Geometry: final body of the model. Coordinates: model frame, mm. Give positions to 0.01 mm unless a question says otherwise; leave off trailing zeros. Loops run counter-clockwise (first coordinate to the right, second up) from the corner with the lowest first, then second, coordinate; pieces in that order, holes last. Notation, with made-up numbers: (61, 5.5) - (81, 5.5) arc R17 cw to (81, 11.5) - close; hole circle Ø10 at (-28.75, 2). An arc over 180 degrees is marked (long way). Use one line per item in the form item = value.
```python
from build123d import *

# Parameters (mm, degrees)
F0_R      = 15.875
F1_DEPTH  = 3.81
F3_DEPTH  = 40.64
F4_DEPTH  = 3.81
F5_DEPTH  = 3.81
F6_DEPTH  = 3.81
F7_DEPTH  = 3.81
F8_DEPTH  = 3.81
F9_DEPTH  = 3.81
F10_DEPTH = 3.81


with BuildPart() as f1:
    # F0 (on Top) → F1 (new body)
    with BuildSketch(Plane.XY):
        with BuildLine():
            Line((-66.04, 50.8), (-88.9, 50.8))
            Line((-88.9, 50.8), (-88.9, 0))
            Line((-88.9, 0), (-69.85, -76.2))
            Line((-69.85, -76.2), (-38.1, -107.95))
            Line((-38.1, -107.95), (0, -107.95))
            Line((0, -107.95), (38.1, -107.95))
            Line((38.1, -107.95), (69.85, -76.2))
            Line((69.85, -76.2), (88.9, 0))
            Line((88.9, 0), (88.9, 50.8))
            Line((88.9, 50.8), (66.04, 50.8))
            Line((66.04, 50.8), (66.04, 1.27))
            Line((66.04, 1.27), (66.04, -36.83))
            Line((66.04, -36.83), (65.8662626902, -36.83))
            ThreePointArc((65.8662626902, -36.83), (47.625, -55.0712626902), (29.3837373098, -36.83))
            Line((29.3837373098, -36.83), (29.21, -36.83))
            Line((29.21, -36.83), (29.21, 1.27))
            Line((29.21, 1.27), (29.21, 50.8))
            Line((29.21, 50.8), (0, 50.8))
            Line((0, 50.8), (-29.21, 50.8))
            Line((-29.21, 50.8), (-29.21, 1.27))
            Line((-29.21, 1.27), (-29.21, -36.83))
            Line((-29.21, -36.83), (-29.3837373098, -36.83))
            ThreePointArc((-29.3837373098, -36.83), (-47.625, -55.0712626902), (-65.8662626902, -36.83))
            Line((-65.8662626902, -36.83), (-66.04, -36.83))
            Line((-66.04, -36.83), (-66.04, 1.27))
            Line((-66.04, 1.27), (-66.04, 50.8))
        make_face()
        with Locations((0, -16.51)):
            Circle(F0_R, mode=Mode.SUBTRACT)
    extrude(amount=F1_DEPTH)

    # F2: F1 across plane


with BuildPart() as f1_1:
    add(f1.part)
    add(f1.part.mirror(Plane.YZ), mode=Mode.INTERSECT)

    # F3 (cut): faces of the model
    f3_faces = [f1_1.faces().sort_by_distance(p)[0] for p in [
        (0, 50.8, 1.905),
        (77.47, 50.8, 1.905),
        (-77.47, 50.8, 1.905),
    ]]
    extrude(f3_faces, amount=-F3_DEPTH, mode=Mode.SUBTRACT)

    # F4 (add): a face of the model
    f4_faces = [f1_1.faces().sort_by_distance(p)[0] for p in [
        (0, -107.95, 1.905),
    ]]
    extrude(f4_faces, amount=F4_DEPTH)

    # F5 (add): a face of the model
    f5_faces = [f1_1.faces().sort_by_distance(p)[0] for p in [
        (-53.975, -92.075, 1.905),
    ]]
    extrude(f5_faces, amount=F5_DEPTH)

    # F6 (add): a face of the model
    f6_faces = [f1_1.faces().sort_by_distance(p)[0] for p in [
        (-79.375, -38.1, 1.905),
    ]]
    extrude(f6_faces, amount=F6_DEPTH)

    # F7 (add): a face of the model
    f7_faces = [f1_1.faces().sort_by_distance(p)[0] for p in [
        (-88.9, 5.08, 1.905),
    ]]
    extrude(f7_faces, amount=F7_DEPTH)

    # F8 (add): a face of the model
    f8_faces = [f1_1.faces().sort_by_distance(p)[0] for p in [
        (53.975, -92.075, 1.905),
    ]]
    extrude(f8_faces, amount=F8_DEPTH)

    # F9 (add): a face of the model
    f9_faces = [f1_1.faces().sort_by_distance(p)[0] for p in [
        (79.375, -38.1, 1.905),
    ]]
    extrude(f9_faces, amount=F9_DEPTH)

    # F10 (add): a face of the model
    f10_faces = [f1_1.faces().sort_by_distance(p)[0] for p in [
        (88.9, 5.08, 1.905),
    ]]
    extrude(f10_faces, amount=F10_DEPTH)


solid = f1_1.part
```
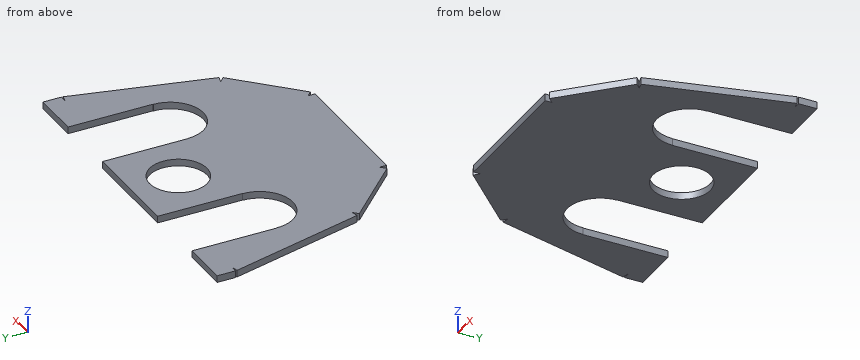
(1) Material intervals for L1, parallel to Y at x = 0, z = 1.85 (3 decimals); L2, parallel to X at y = -16.51, z = 1.65 (3 decimals); L3, parallel to X at y = -11, z = 1.8, sorted ascending. Write a range as from..to.
Solution:
L1 = -111.76..-32.385, -0.635..10.16
L2 = -88.7..-66.04, -29.21..-15.875, 15.875..29.21, 66.04..88.7
L3 = -90.08..-66.04, -29.21..-14.89, 14.89..29.21, 66.04..90.08
(2) Cut plane D-D (y = -39). Return the cut outline in (x, z).
Solution:
outline = (-83.08, 0) - (-65.74, 0) - (-65.74, 3.81) - (-83.08, 3.81) - close; (-29.51, 0) - (29.51, 0) - (29.51, 3.81) - (-29.51, 3.81) - close; (65.74, 0) - (83.08, 0) - (83.08, 3.81) - (65.74, 3.81) - close
(3) Cut plane B-B (x = -12). Return the cut outline in (y, z), plus the area to 3 significant figures.
Solution:
outline = (-111.76, 0) - (-26.9, 0) - (-26.9, 3.81) - (-111.76, 3.81) - close; (-6.12, 0) - (10.16, 0) - (10.16, 3.81) - (-6.12, 3.81) - close
area = 385 mm2
(4) Cut plane C-C (y = -21.5). Return the cut outline in (x, z), plus the area to 3 significant figures.
Solution:
outline = (-87.45, 0) - (-66.04, 0) - (-66.04, 3.81) - (-87.45, 3.81) - close; (-29.21, 0) - (-15.07, 0) - (-15.07, 3.81) - (-29.21, 3.81) - close; (15.07, 0) - (29.21, 0) - (29.21, 3.81) - (15.07, 3.81) - close; (66.04, 0) - (87.45, 0) - (87.45, 3.81) - (66.04, 3.81) - close
area = 271 mm2
(5) Pin query (flat end, axial travel): P1, Ø1.9, axis at y = -110, z = 2, coming from the +X side; P2, Ø1.5, axis at y = -19, z = 0.5, coming from the -X side; P3, Ø1.9, axis at y = -3.5, z = 1, coming from the -X side. Return the tip coordinate at first contact, or that it passes through.
Solution:
P1 = 42.39
P2 = -88.26
P3 = -92.19
